Study the drawing (mm; zero at the part's minimum x, y, z) and answer. Give positions to 0.01 mm unless a question says otherwise; leave off trailing zeros. Write each loop counter-clockwise with the first axis right and the second up, starting at its lowest first coordinate (ties: lowest second). Pieces come first, ordered by that corner, then holes.
1) A straight line is drawn through the part: probe 1 along X at (y, z) = (11.5, 15). Find the intervals that lie inside material, in ascending order.
2) Find section B-B (y = 16.25). Determine the outline of the cut face in (x, z), plus the area to 3 significant figures.
3) Find section A-A (z = 15). Determine the outline of the cut face in (x, y), plus the area to 4 significant figures.
4) Find section C-C (x = 15). Determine the outline of the cut face in (y, z).
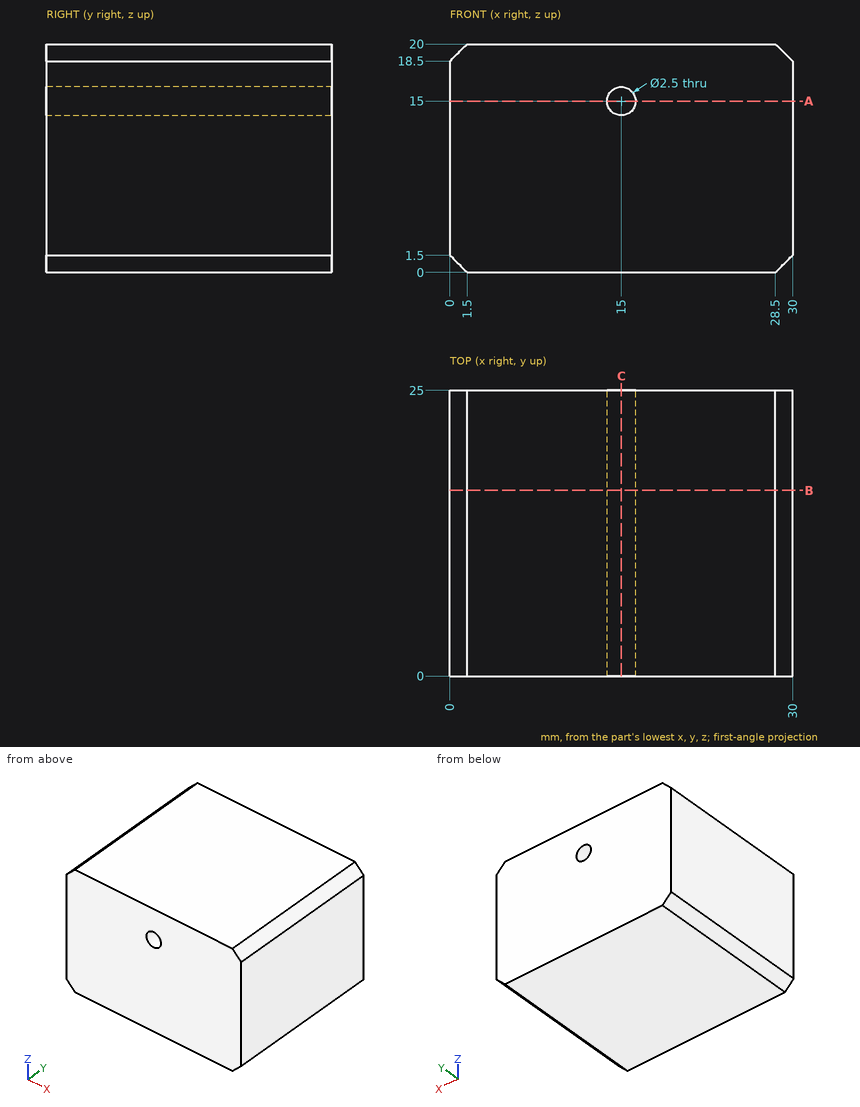
Results:
1. probe 1: x = 0 to 13.75, 16.25 to 30
2. outline: (0, 1.5) - (1.5, 0) - (28.5, 0) - (30, 1.5) - (30, 18.5) - (28.5, 20) - (1.5, 20) - (0, 18.5) - close; hole circle Ø2.5 at (15, 15)
2. area: 591 mm2
3. outline: (0, 0) - (13.75, 0) - (13.75, 25) - (0, 25) - close; (16.25, 0) - (30, 0) - (30, 25) - (16.25, 25) - close
3. area: 687.5 mm2
4. outline: (0, 0) - (25, 0) - (25, 13.75) - (0, 13.75) - close; (0, 16.25) - (25, 16.25) - (25, 20) - (0, 20) - close
